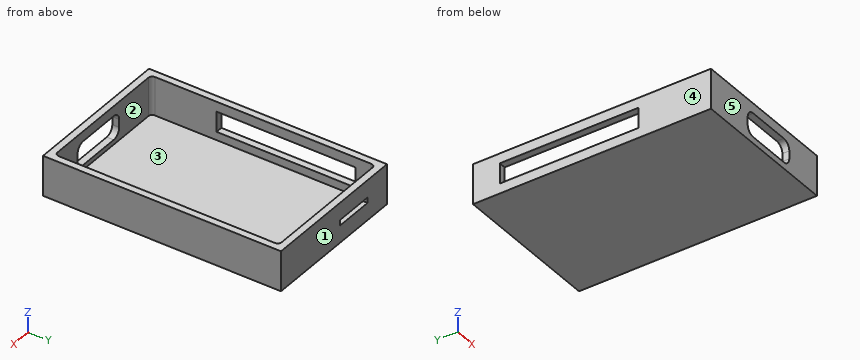
```python
from build123d import *

# Parameters (mm, degrees)
SKETCH_1_W          = 76.5
SKETCH_1_H          = 120
EXTRUDE_1_DEPTH     = 0.8
SKETCH_10_W         = 76.5
SKETCH_10_H         = 120
SKETCH_10_W_2       = 69.5
SKETCH_10_H_2       = 113
EXTRUDE_2_DEPTH     = 19.4
FILLET_1_R          = 2
SKETCH_11_W         = 10.2
SKETCH_11_H         = 70
CUT_EXTRUDE_1_DEPTH = 3.5
SKETCH_12_W         = 30
SKETCH_12_H         = 12
CUT_EXTRUDE_2_DEPTH = 10
FILLET_2_R          = 4
CUT_EXTRUDE_3_REACH = 122
SKETCH_13_W         = 20
SKETCH_13_H         = 2.8


with BuildPart() as part:
    # ｽｹｯﾁ1 → ﾎﾞｽ - 押し出し1 (new body)
    with BuildSketch(Plane.XY):
        with Locations((38.25, 60)):
            Rectangle(SKETCH_1_W, SKETCH_1_H)
    extrude(amount=EXTRUDE_1_DEPTH)

    # ｽｹｯﾁ10 → ﾎﾞｽ - 押し出し2 (add)
    with BuildSketch(Plane.XY.offset(0.8)):
        with Locations((38.25, 60)):
            Rectangle(SKETCH_10_W, SKETCH_10_H)
        with Locations((38.25, 60)):
            Rectangle(SKETCH_10_W_2, SKETCH_10_H_2, mode=Mode.SUBTRACT)
    extrude(amount=EXTRUDE_2_DEPTH)

    # ﾌｨﾚｯﾄ1
    fillet_1_edges = [part.edges().sort_by_distance(p)[0] for p in [
        (73, 116.5, 10.5),
        (3.5, 116.5, 10.5),
        (3.5, 3.5, 10.5),
        (73, 3.5, 10.5),
    ]]
    fillet(fillet_1_edges, radius=FILLET_1_R)

    # ｽｹｯﾁ11 → ｶｯﾄ - 押し出し1 (cut)
    with BuildSketch(Plane.ZY):
        with Locations((10.1, 71.5)):
            Rectangle(SKETCH_11_W, SKETCH_11_H)
    extrude(amount=-CUT_EXTRUDE_1_DEPTH, mode=Mode.SUBTRACT)

    # ｽｹｯﾁ12 → ｶｯﾄ - 押し出し2 (cut)
    with BuildSketch(Plane(origin=(0, 0, 0), x_dir=(-1, 0, 0), z_dir=(0, -1, 0))):
        with Locations((-41.5, -9.2)):
            Rectangle(SKETCH_12_W, SKETCH_12_H)
    extrude(amount=-CUT_EXTRUDE_2_DEPTH, mode=Mode.SUBTRACT)

    # ﾌｨﾚｯﾄ2
    fillet_2_edges = [part.edges().sort_by_distance(p)[0] for p in [
        (56.5, 1.75, 15.2),
        (56.5, 1.75, 3.2),
        (26.5, 1.75, 3.2),
        (26.5, 1.75, 15.2),
    ]]
    fillet(fillet_2_edges, radius=FILLET_2_R)

    # ｽｹｯﾁ13 → ｶｯﾄ - 押し出し3 (cut, up to next)
    with BuildSketch(Plane(origin=(0, 120, 0), x_dir=(1, 0, 0), z_dir=(0, 1, 0)), mode=Mode.PRIVATE) as cut_extrude_3_sk1:
        with Locations((24, -10.1)):
            Rectangle(SKETCH_13_W, SKETCH_13_H)
    cut_extrude_3_tool1 = extrude(cut_extrude_3_sk1.sketch, amount=-CUT_EXTRUDE_3_REACH, mode=Mode.PRIVATE) & part.part
    add(cut_extrude_3_tool1.solids().sort_by_distance((24, 120, 10.1))[0], mode=Mode.SUBTRACT)


solid = part.part
```
Build history of the part. All positions in model axes, mm. Face numbers are marked on the shaded views. A direction names the side the tool comes from. Round coordinates to 2 decimals unless told otherwise and drop trailing zeros. Loops run counter-clockwise (first coordinate to the right, second up) from the corner with the lowest first, then second, coordinate; pieces in that order, holes last.
Item 1: Which spindle directions (+Z, -Z, +X, -X, +Y, -Y) get a long thin tool onto all of the face, cutting with end or side? Do the marked faces 1 and 2. Say none if no direction does.
Item 2: Pin check, flat tips, straight feed: P1, Ø5, axis at x = 47.5, z = 12, coming from the -Y side; P2, Ø10, axis at x = 43.5, y = 93, coming from the +Z side. Stop position of each tip, or through.
Item 3: Saw through at C-C (z = 12.75). List the corners of the cut face in (x, y), then the cut area to 3 significant figures.
Item 4: Saw through at B-B (x = 39). List the corners of the cut face in (y, z), then the cut area to 3 significant figures.
Item 5: Saw through at A-A (y = 39.5). List the corners of the cut face in (x, z), then the cut area to 3 significant figures.
Item 6: Two-plate mould, pull along Y, no slides. Class the marked faces 3, 4 and 5: released by +Y, released by -Y, zero draft, split by the parting line, or undercut.
Item 7: Saw through at D-D (x = 63). List the corners of the cut face in (y, z), then the cut area to 3 significant figures.
Item 8: Drill centre lines: line 1 along Y through (x, z) = (39.5, 16.5); line 2 along X through (y, z) = (32.5, 11.5); line 3 along X through (y, z) = (82.5, 11.5). Where is each one in solid material? Low to high.
Worked answers:
1. face 1: +Z, -Z, +X, -X, +Y
1. face 2: +Z
2. P1: stops at y = 116.5
2. P2: stops at z = 0.8
3. outline: (0, 0) - (26.81, 0) - (26.81, 3.5) - (5.5, 3.5) arc R2 cw to (3.5, 5.5) - (3.5, 36.5) - (0, 36.5) - close; (0, 106.5) - (3.5, 106.5) - (3.5, 114.5) arc R2 cw to (5.5, 116.5) - (71, 116.5) arc R2 cw to (73, 114.5) - (73, 5.5) arc R2 cw to (71, 3.5) - (56.19, 3.5) - (56.19, 0) - (76.5, 0) - (76.5, 120) - (0, 120) - close
3. area: 982 mm2
4. outline: (0, 0) - (120, 0) - (120, 20.2) - (116.5, 20.2) - (116.5, 0.8) - (3.5, 0.8) - (3.5, 3.2) - (0, 3.2) - close; (0, 15.2) - (3.5, 15.2) - (3.5, 20.2) - (0, 20.2) - close
4. area: 190 mm2
5. outline: (0, 0) - (76.5, 0) - (76.5, 20.2) - (73, 20.2) - (73, 0.8) - (3.5, 0.8) - (3.5, 5) - (0, 5) - close; (0, 15.2) - (3.5, 15.2) - (3.5, 20.2) - (0, 20.2) - close
5. area: 161 mm2
6. face 3: undercut
6. face 4: zero draft
6. face 5: released by -Y
7. outline: (0, 0) - (120, 0) - (120, 20.2) - (116.5, 20.2) - (116.5, 0.8) - (3.5, 0.8) - (3.5, 20.2) - (0, 20.2) - close
7. area: 232 mm2
8. line 1: y = 0 to 3.5, 116.5 to 120
8. line 2: x = 0 to 3.5, 73 to 76.5
8. line 3: x = 73 to 76.5
